Input: part model. Units: mm. Frame: model coordinates. A direction names the side the tool comes from. Coordinates: 2 decimals unless noted, no trailing zeros. Loops run counter-clockwise (first coordinate to the right, second up) from the corner with the lowest first, then second, coordinate; pieces in that order, holes last.
Item 1: Reachability of faces 1 (the flat face through (-1.5, 46, 1)), 2 (the flat face through (1.5, 45, 1)), 3 (the flat face through (0, 32, 0)) from +Z, -Z, +X, -X, +Y, -Y: full face, straight path, thin tool, end or side. Return the list, or none.
Item 2: Section B-B on y = 60.5. Return loops of the section in (x, z), and give its area (3 significant figures).
Item 3: Pull-direction query (X, two-part tool) for faces 4 (the cylindrical face through (1.35, 0.42, 0.74)), 5 (the flat face through (0, 32, 1.5)), 6 (the cylindrical face through (0, -6, 1)); classes: released by +X, released by -X, zero draft, split by the parting line, or undercut.
Item 4: Ray query, line 1 along X through (y, z) = (59.5, 0.85); line 2 along Y through (x, z) = (0.5, 1.3); line 3 along X through (y, z) = (86, 0.25). Return the intervals inside material, ascending.
Item 5: Section A-A on y = 0. Return loops of the section in (x, z).
Item 6: Contact query for a flat-ended pin moving along its axis: P1, Ø0.8, axis at y = 32.5, z = 0.5, coming from the +X side. Output: stop coordinate, or through.
Item 7: Section C-C on x = -3. Return loops of the section in (y, z).
```python
from build123d import *

# Parameters (mm, degrees)
SKETCH2_R           = 1.412460089
BOSS_EXTRUDE1_DEPTH = 1.5


with BuildPart() as part:
    # Sketch2 → Boss-Extrude1 (new body)
    with BuildSketch(Plane.XY):
        with BuildLine():
            Line((-1.5, 85.125143236), (-1.5, 5.809475019))
            ThreePointArc((-1.5, 5.809475019), (0, -6), (1.5, 5.809475019))
            Line((1.5, 5.809475019), (1.5, 85.125143236))
            add(Edge.make_bspline(
                [(0, 90), (1.319809251, 87.72856759), (1.5, 85.125143236)],
                knots=[0, 0, 0, 1, 1, 1], degree=2))
            add(Edge.make_bspline(
                [(0, 90), (-1.319809251, 87.72856759), (-1.5, 85.125143236)],
                knots=[0, 0, 0, 1, 1, 1], degree=2))
        make_face()
        Circle(SKETCH2_R, mode=Mode.SUBTRACT)
    extrude(amount=BOSS_EXTRUDE1_DEPTH)


solid = part.part
```
Results found:
1. face 1: +Z, -Z, -X, +Y
1. face 2: +Z, -Z, +X, +Y
1. face 3: -Z, +X, -X, +Y, -Y
2. outline: (-1.5, 0) - (1.5, 0) - (1.5, 1.5) - (-1.5, 1.5) - close
2. area: 4.50 mm2
3. face 4: undercut
3. face 5: zero draft
3. face 6: split by the parting line
4. line 1: x = -1.5 to 1.5
4. line 2: y = -5.98 to -1.32, 1.32 to 89.04
4. line 3: x = -1.41 to 1.41
5. outline: (-6, 0) - (-1.41, 0) - (-1.41, 1.5) - (-6, 1.5) - close; (1.41, 0) - (6, 0) - (6, 1.5) - (1.41, 1.5) - close
6. P1: stops at x = 1.5
7. outline: (-5.2, 0) - (5.2, 0) - (5.2, 1.5) - (-5.2, 1.5) - close
